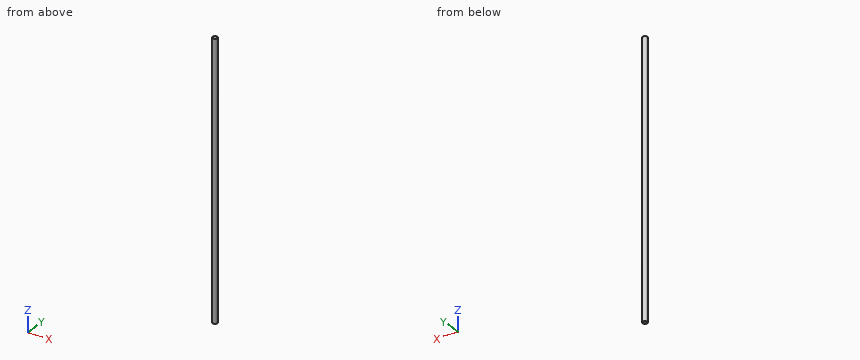
```python
from build123d import *

# Parameters (mm, degrees)
SKETCH1_R           = 4
EXTRUDE2_DEPTH      = 225
EXTRUDE2_DEPTH_BACK = 225
FILLET2_R           = 1
FILLET3_R           = 1


with BuildPart() as part:
    # Sketch1 → Extrude2 (new body, two sides)
    with BuildSketch(Plane.XY) as extrude2_sk:
        Circle(SKETCH1_R)
    extrude(amount=EXTRUDE2_DEPTH)
    extrude(extrude2_sk.sketch, amount=-EXTRUDE2_DEPTH_BACK)

    # Fillet2
    fillet2_edges = [part.edges().sort_by_distance(p)[0] for p in [
        (-4, 0, -225),
    ]]
    fillet(fillet2_edges, radius=FILLET2_R)

    # Fillet3
    fillet3_edges = [part.edges().sort_by_distance(p)[0] for p in [
        (-4, 0, 225),
    ]]
    fillet(fillet3_edges, radius=FILLET3_R)


solid = part.part
```
Work out the finished part from the listing and answer in its coordinate system (mm). Round coordinates to 2 decimals unless told otherwise and drop trailing zeros. Write each loop counter-clockwise with the first axis right and the second up, starting at its lowest first coordinate (ties: lowest second). Pieces come first, ordered by that corner, then holes.
1) Flat-ended cylindrical pins translate along their axes: P1, Ø4, axis at x = 2.5, z = -50.5, coming from the +Y side; P2, Ø1, axis at x = 3, y = 2, coming from the +Z side; P3, Ø2, axis at x = 1.5, z = -96, coming from the -Y side. Find the tip coordinate at first contact, or state that the pin passes through.
2) A cutting plane is placed at A-A on z = 164. Determine the outline of the cut face in (x, y).
3) Consider probe 1 along Y at (x, z) = (0.75, 69.5); probe 2 along X at (y, z) = (0.25, -26.5). Determine where each line is inside the solid, lowest interval first.
Entries:
1. P1: stops at y = 3.97
1. P2: stops at z = 224.99
1. P3: stops at y = -3.97
2. outline: circle Ø8 at (0, 0)
3. probe 1: y = -3.93 to 3.93
3. probe 2: x = -3.99 to 3.99
